Source: three-view drawing plus pictorial views. Frame: mm from the lowest corner of the part. A direction names the side the tool comes from. Give positions to 0.01 mm unless a question says otherwise; leave off trailing zeros. Order: outer loops, then holes, each group sorted by start corner. A loop starts at its lowest first (then second) coordinate and runs counter-clockwise, first axis right, second up.
1) First-contact query: P1, Ø7, axis at x = 97.5, y = 11, coming from the +Z side. Flat tip, straight axial feed; report the tip coordinate or a pass-through.
2) Section B-B, the plane x = 118. Return loops of the section in (y, z), plus the area to 3 significant figures.
3) Section D-D, the plane z = 22.5. Return loops of the section in (x, y), plus the area to 3 significant figures.
4) Draft query along X for the marked faces 3, 4 and 5. Return one class per face: released by +X, released by -X, zero draft, split by the parting line, or undercut.
5) Access query for the marked faces 1 and 2. Directions: +Z, -Z, +X, -X, +Y, -Y. A direction counts if a zero-diameter tool reaches every point of the face in a straight line with its end or side. Return the directions, or none.
6) Section C-C, the plane y = 1.5. Return loops of the section in (x, z), plus the area to 3 significant figures.
7) Section A-A, the plane x = 32.5. Return loops of the section in (y, z).
8) Material intervals for line 1 (Z direction, x = 118, y = 9.25); line 2 (Y direction, x = 59.5, z = 20.25); line 3 (X direction, y = 15, z = 22.5), sorted ascending.
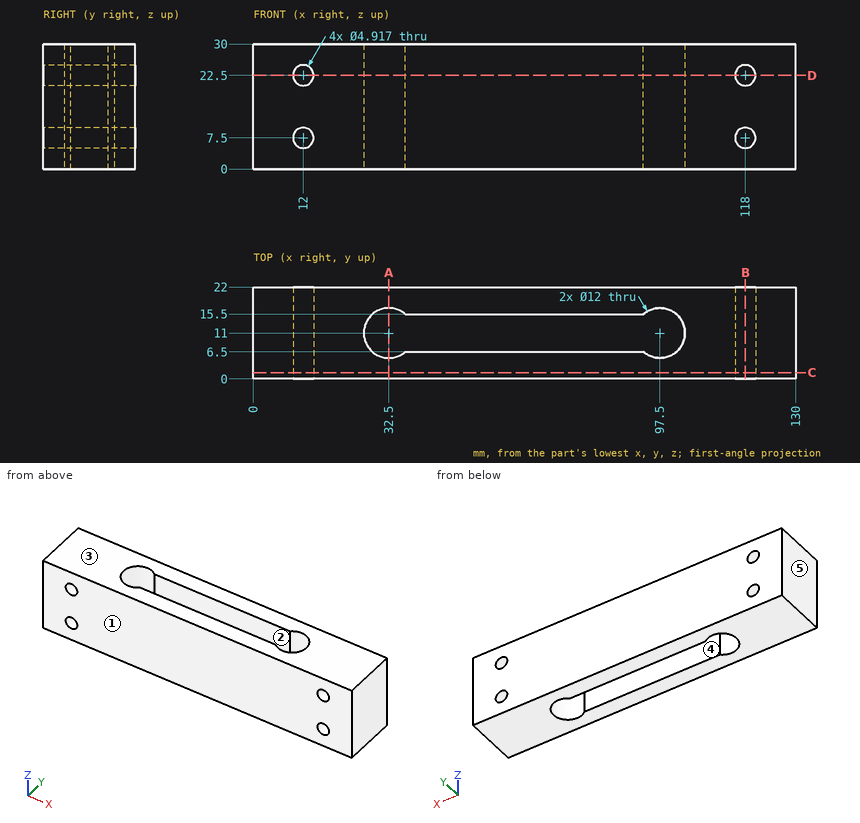
From the geometry:
1. P1: passes through
2. outline: (0, 0) - (22, 0) - (22, 5.04) - (0, 5.04) - close; (0, 9.96) - (22, 9.96) - (22, 20.04) - (0, 20.04) - close; (0, 24.96) - (22, 24.96) - (22, 30) - (0, 30) - close
2. area: 444 mm2
3. outline: (0, 0) - (9.54, 0) - (9.54, 22) - (0, 22) - close; (14.46, 0) - (115.54, 0) - (115.54, 22) - (14.46, 22) - close; (120.46, 0) - (130, 0) - (130, 22) - (120.46, 22) - close; hole (36.47, 6.5) - (93.53, 6.5) arc R6 ccw (long way) to (93.53, 15.5) - (36.47, 15.5) arc R6 ccw (long way) to start
3. area: 1,930 mm2
4. face 3: zero draft
4. face 4: undercut
4. face 5: released by -X
5. face 1: +Z, -Z, +X, -X, -Y
5. face 2: +Z, -Z
6. outline: (0, 0) - (130, 0) - (130, 30) - (0, 30) - close; hole circle Ø4.92 at (12, 7.5); hole circle Ø4.92 at (12, 22.5); hole circle Ø4.92 at (118, 7.5); hole circle Ø4.92 at (118, 22.5)
6. area: 3,820 mm2
7. outline: (0, 0) - (5, 0) - (5, 30) - (0, 30) - close; (17, 0) - (22, 0) - (22, 30) - (17, 30) - close
8. line 1: z = 0 to 5.04, 9.96 to 20.04, 24.96 to 30
8. line 2: y = 0 to 6.5, 15.5 to 22
8. line 3: x = 0 to 9.54, 14.46 to 28.03, 101.97 to 115.54, 120.46 to 130
